Verification items for the finished model (mm, model axes). Round coordinates to 2 decimals unless told otherwise and drop trailing zeros. Loops run counter-clockwise (first coordinate to the right, second up) from the corner with the lowest first, then second, coordinate; pieces in that order, holes last. Notation, with made-up numbers: M 40.25,-28 L 55.25,-28 A18 ccw 55.25,-15 Z; hole C 3.5,12 d3. An arc over 180 degrees is marked long. One line per item, written item: value.
from build123d import *

# Parameters (mm, degrees)
F0_W     = 194
F0_H     = 50
F1_DEPTH = 3
F2_W     = 3
F2_H     = 5
F3_DEPTH = 3
F4_R     = 8
F5_DEPTH = 25


with BuildPart() as f1:
    # F0 (on Front) → F1 (new body)
    with BuildSketch(Plane.XZ):
        Rectangle(F0_W, F0_H)
    extrude(amount=F1_DEPTH)

    # F2 (on face) → F3 (join)
    with BuildSketch(Plane.XZ.offset(3)):
        with Locations((-98.5, 22.5)):
            Rectangle(F2_W, F2_H)
        with Locations((-98.5, 12.5)):
            Rectangle(F2_W, F2_H)
        with Locations((-98.5, 2.5)):
            Rectangle(F2_W, F2_H)
        with Locations((-98.5, -7.5)):
            Rectangle(F2_W, F2_H)
        with Locations((-98.5, -17.5)):
            Rectangle(F2_W, F2_H)
        with Locations((98.5, 12.5)):
            Rectangle(F2_W, F2_H)
        with Locations((98.5, 22.5)):
            Rectangle(F2_W, F2_H)
        with Locations((98.5, 2.5)):
            Rectangle(F2_W, F2_H)
        with Locations((98.5, -7.5)):
            Rectangle(F2_W, F2_H)
        with Locations((98.5, -17.5)):
            Rectangle(F2_W, F2_H)
    extrude(amount=-F3_DEPTH)

    # F4 (on face) → F5 (cut)
    with BuildSketch(Plane.XZ.offset(3)):
        with Locations((-72, -5)):
            Circle(F4_R)
        with Locations((72, -5)):
            Circle(F4_R)
    extrude(amount=-F5_DEPTH, mode=Mode.SUBTRACT)


solid = f1.part
(1) Sectioned sample at B-B on y = -2.4. Count the separate pieces of the cut face and the enclosed holes in it, and give its area (3 significant figures).
Completed:
separate pieces: 1
enclosed holes: 2
area: 9,450 mm^2
(2) Mould release check, pull along Z, two halves, no side actions. Record for faces 1 (the face through (65.651, -1.521, -9.868)), 2 (the face through (-1, 0, 0)): +Z half, -Z half, draft (parallel to the pull), parting line (faces both ways), or undercut.
Completed:
face 1: undercut
face 2: draft
(3) Depth check by flat-ended pin: pin 1 Ø1.5 at (x, y) = (98.5, -1.5) entering from -Z; pin 2 Ø1.5 at (y, z) = (-2, -1.5) entering from -X. Enter the tip coordinate at first touch or a pass-through.
Completed:
pin 1: stops at z = -20
pin 2: stops at x = -97
(4) Sectioned sample at A-A on x = 72. Enter the section's corners in (y, z).
Completed:
outline: M -3,-25 L 0,-25 L 0,-13 L -3,-13 Z; M -3,3 L 0,3 L 0,25 L -3,25 Z
(5) Thickness scan on L1, parallel to Z at x = 72, y = -1.05; L2, parallel to X at y = -1.4, z = 6; L3, parallel to X at y = -1, z = -1.5. Record the ranges inside material, lowest first. Write a range as from..to.
Completed:
L1: z = -25..-13, 3..25
L2: x = -97..97
L3: x = -97..-79.19, -64.81..64.81, 79.19..97
